For this review, take the finished solid that the model builds, in its own axes (mm). Face numbers are marked on the shaded views. A direction names the side the tool comes from. Give positions to 0.01 mm unless a question says otherwise; leave off trailing zeros. Loops run counter-clockwise (first coordinate to the right, second up) from the corner with the lowest first, then second, coordinate; pieces in that order, holes last.
```python
from build123d import *

# Parameters (mm, degrees)
F0_W      = 57.8200779855
F0_H      = 67.2501921654
F1_DEPTH  = 25.4
F2_W      = 57.8200779855
F2_H      = 17.7068114281
F3_DEPTH  = 83.566
F4_W      = 19.4322280586
F4_H      = 20.8092816174
F5_DEPTH  = 43.688
F6_R      = 9.7161140293
F7_DEPTH  = 25.4
F9_DEPTH  = 16.764
F10_R     = 28.9100389928
F11_DEPTH = 25.4


with BuildPart() as f1:
    # F0 (on Top) → F1 (new body)
    with BuildSketch(Plane.XY):
        Rectangle(F0_W, F0_H)
    extrude(amount=F1_DEPTH)

    # F2 (on face) → F3 (join)
    with BuildSketch(Plane.XY.offset(25.4)):
        with Locations((0, 24.7716903687)):
            Rectangle(F2_W, F2_H)
    extrude(amount=F3_DEPTH)

    # F4 (on face) → F5 (cut)
    with BuildSketch(Plane.XY.offset(108.966)):
        with Locations((0, 26.3229254633)):
            Rectangle(F4_W, F4_H)
    extrude(amount=-F5_DEPTH, mode=Mode.SUBTRACT)

    # F6 (on face) → F7 (cut)
    with BuildSketch(Plane.XZ.offset(-15.9182846546)):
        with Locations((0, 65.278)):
            Circle(F6_R)
    extrude(amount=-F7_DEPTH, mode=Mode.SUBTRACT)

    # F8 (on face) → F9 (cut)
    with BuildSketch(Plane.YZ.offset(28.9100389928)):
        Polygon((15.9182846546, 25.4), (0, 25.4), (0, 0), (33.6250960827, 0), (33.6250960827, 37.1936224401), (15.9182846546, 37.1936224401), align=None)
    extrude(amount=-F9_DEPTH, mode=Mode.SUBTRACT)

    # F10 (on face) → F11 (join)
    with BuildSketch(Plane(origin=(0, 0, 0), x_dir=(1, 0, 0), z_dir=(0, 0, -1))):
        with Locations((0, 33.6250960827)):
            Circle(F10_R)
    extrude(amount=-F11_DEPTH)


solid = f1.part
```
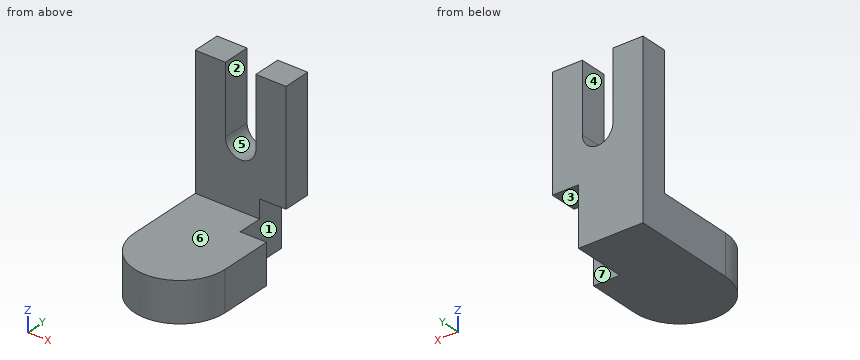
Item 1: Take a section at C-C on x = 0. Give the boundary of the cut face in (y, z).
Answer:
outline: (-62.54, 0) - (33.63, 0) - (33.63, 55.56) - (15.92, 55.56) - (15.92, 25.4) - (-62.54, 25.4) - close
Item 2: Tool access review of the marked faces 5, 6 and 7: name each direction out of +Z, -Z, +X, -X, +Y, -Y from which nothing blocks a thin tool from reaching the whole face with its end or side.
Answer:
face 5: +Z, +Y, -Y
face 6: +Z, +X, -X, -Y
face 7: +Z, -Z, +X, +Y
Item 3: Clearance check with flat-ended pins moving along their axes: pin 1 Ø2 at (x, y) = (-16, -10.5) entering from +Z; pin 2 Ø5 at (x, z) = (-17.5, 21.5) entering from -Y; pin 3 Ø5 at (x, y) = (0.5, -15) entering from -Z; pin 4 Ø8.5 at (x, y) = (18, 23) entering from -Z. State where each tip first meets the part, or that it passes through.
Answer:
pin 1: stops at z = 25.4
pin 2: stops at y = -58.34
pin 3: stops at z = 0
pin 4: stops at z = 37.19
Item 4: Take a section at D-D on z = 21. Give the boundary of the cut face in (x, y), and give its area (3 significant figures).
Answer:
outline: (-28.91, -33.63) arc R28.91 ccw to (28.91, -33.63) - (28.91, 0) - (12.15, 0) - (12.15, 33.63) - (-28.91, 33.63) - close
area: 4,640 mm2
Item 5: Take a section at B-B on x = 18. Give the boundary of the cut face in (y, z).
Answer:
outline: (-56.25, 0) - (0, 0) - (0, 25.4) - (-56.25, 25.4) - close; (15.92, 37.19) - (33.63, 37.19) - (33.63, 108.97) - (15.92, 108.97) - close
Item 6: For L1, parallel to Y at x = 17, z = 39.5; L2, parallel to Z at x = -20, y = -52.5; L3, parallel to X at y = 8, z = 20.5, list the stretches that pass through material, from the lowest coordinate up.
Answer:
L1: y = 15.92 to 33.63
L2: z = 0 to 25.4
L3: x = -28.91 to 12.15
Item 7: The part is to be moulded in two halves that separate along X. For the marked faces 1, 2, 3 and 4, say which applies: released by +X, released by -X, zero draft, split by the parting line, or undercut.
Answer:
face 1: released by +X
face 2: undercut
face 3: zero draft
face 4: undercut
Item 8: Take a section at A-A on z = 97. Give the boundary of the cut face in (x, y).
Answer:
outline: (-28.91, 15.92) - (-9.72, 15.92) - (-9.72, 33.63) - (-28.91, 33.63) - close; (9.72, 15.92) - (28.91, 15.92) - (28.91, 33.63) - (9.72, 33.63) - close
